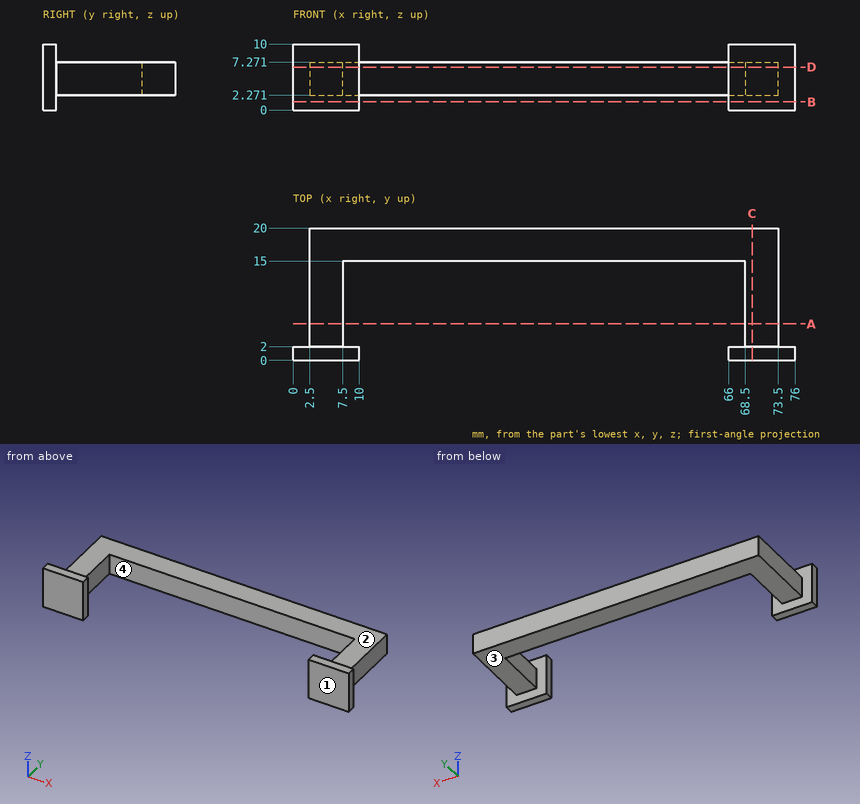
Source: three-view drawing plus pictorial views. Frame: mm from the lowest corner of the part. A direction names the side the tool comes from. Round coordinates to 2 decimals unless told otherwise and drop trailing zeros. Loops run counter-clockwise (first coordinate to the right, second up) from the corner with the lowest first, then second, coordinate; pieces in that order, holes last.
1. Section query B-B on z = 1.25. Output: boundary loops of the cut face in (x, y), and give its area (3 significant figures).
2. Contact query for flat-ended pins moving along their axis: pin 1 (1.5 mm diameter, centred on x = 60.5, y = 18, fed in from -Z); pin 2 (6 mm diameter, centred on x = 42.5, y = 17, fed in from +Z); pin 3 (1.5 mm diameter, centred on y = 10.5, z = 5.5, fed in from +X); pin 4 (9 mm diameter, centred on x = 25, y = 7.5, fed in from +Z). Output: stop coordinate, or through.
3. Section query D-D on z = 6.5. Output: boundary loops of the cut face in (x, y).
4. Mould query, pull axis X, two halves, no side actions, for the marked faces 3 and 4. Classes: released by +X, released by -X, zero draft, split by the parting line, or undercut.
5. Section query C-C on x = 69.5. Output: boundary loops of the cut face in (y, z).
6. Section query A-A on y = 5.5. Output: boundary loops of the cut face in (x, z).
7. Ray query, L1, parallel to X at y = 8.5, z = 3.75; L2, parallel to Y at x = 8.5, z = 3.75; L3, parallel to Y at x = 19, z = 6.25. Return the intervals inside material, ascending.
8. Access query for the marked faces 1 and 2. Directions: +Z, -Z, +X, -X, +Y, -Y. A direction counts if a zero-diameter tool reaches every point of the face in a straight line with its end or side. Return the directions, or none.
Answers below:
1. outline: (0, 0) - (10, 0) - (10, 2) - (0, 2) - close; (66, 0) - (76, 0) - (76, 2) - (66, 2) - close
1. area: 40.0 mm2
2. pin 1: stops at z = 2.27
2. pin 2: stops at z = 7.27
2. pin 3: stops at x = 73.5
2. pin 4: passes through
3. outline: (0, 0) - (10, 0) - (10, 2) - (7.5, 2) - (7.5, 15) - (68.5, 15) - (68.5, 2) - (66, 2) - (66, 0) - (76, 0) - (76, 2) - (73.5, 2) - (73.5, 20) - (2.5, 20) - (2.5, 2) - (0, 2) - close
4. face 3: zero draft
4. face 4: undercut
5. outline: (0, 0) - (2, 0) - (2, 2.27) - (20, 2.27) - (20, 7.27) - (2, 7.27) - (2, 10) - (0, 10) - close
6. outline: (2.5, 2.27) - (7.5, 2.27) - (7.5, 7.27) - (2.5, 7.27) - close; (68.5, 2.27) - (73.5, 2.27) - (73.5, 7.27) - (68.5, 7.27) - close
7. L1: x = 2.5 to 7.5, 68.5 to 73.5
7. L2: y = 0 to 2, 15 to 20
7. L3: y = 15 to 20
8. face 1: +Z, -Z, +X, -X, -Y
8. face 2: +Z, +X, -X, +Y
